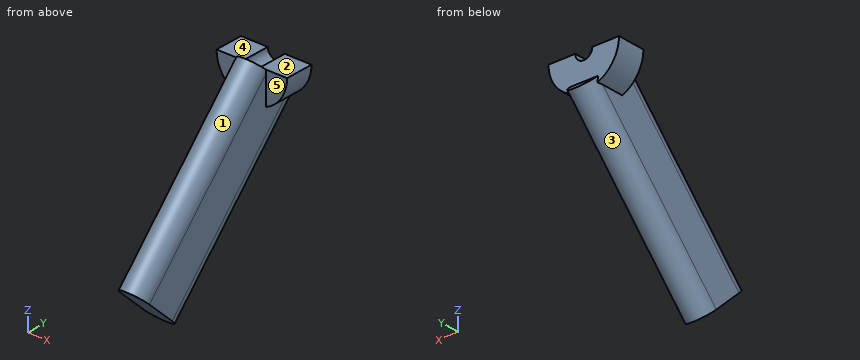
```python
from build123d import *

# Parameters (mm, degrees)
F1_DEPTH = 25
F5_DEPTH = 176


with BuildPart() as f1:
    # F0 (on Front) → F1 (new body)
    with BuildSketch(Plane.XZ):
        with BuildLine():
            ThreePointArc((-31, 0), (0, -31), (31, 0))
            Line((31, 0), (7.5, 0))
            ThreePointArc((7.5, 0), (0, -7.5), (-7.5, 0))
            Line((-7.5, 0), (-31, 0))
        make_face()
    extrude(amount=F1_DEPTH)

    # F4 (on face) → F5 (join)
    with BuildSketch(Plane(origin=(0, -11.816696451, -12.4813098776), x_dir=(1, 0, 0), z_dir=(0, -0.6875084422, -0.7261763849))):
        with BuildLine():
            Line((-12.5, 16), (0, 16))
            Line((0, 16), (12.5, 16))
            ThreePointArc((12.5, 16), (0, 28.5), (-12.5, 16))
        make_face()
        with BuildLine():
            Line((0, 16), (0, 3.5))
            ThreePointArc((0, 3.5), (8.8388347648, 7.1611652352), (12.5, 16))
            Line((12.5, 16), (0, 16))
        make_face()
        with BuildLine():
            ThreePointArc((-12.5, 16), (-8.8388347648, 7.1611652352), (0, 3.5))
            Line((0, 3.5), (0, 16))
            Line((0, 16), (-12.5, 16))
        make_face()
        with BuildLine():
            Line((0, -16), (0, -3.5))
            ThreePointArc((0, -3.5), (-8.8388347648, -7.1611652352), (-12.5, -16))
            ThreePointArc((-12.5, -16), (0, -28.5), (12.5, -16))
            Line((12.5, -16), (0, -16))
        make_face()
        with BuildLine():
            Line((0, 3.5), (0, 0))
            Line((0, 0), (0, -3.5))
            ThreePointArc((0, -3.5), (8.8388347648, -7.1611652352), (12.5, -16))
            Line((12.5, -16), (12.5, 16))
            ThreePointArc((12.5, 16), (8.8388347648, 7.1611652352), (0, 3.5))
        make_face()
        with BuildLine():
            Line((0, -3.5), (0, 0))
            Line((0, 0), (0, 3.5))
            ThreePointArc((0, 3.5), (-8.8388347648, 7.1611652352), (-12.5, 16))
            Line((-12.5, 16), (-12.5, -16))
            ThreePointArc((-12.5, -16), (-8.8388347648, -7.1611652352), (0, -3.5))
        make_face()
        with BuildLine():
            ThreePointArc((12.5, -16), (8.8388347648, -7.1611652352), (0, -3.5))
            Line((0, -3.5), (0, -16))
            Line((0, -16), (12.5, -16))
        make_face()
    extrude(amount=F5_DEPTH)


solid = f1.part
```
Could you check a few things on this model? Use its own coordinates, in mm. Face numbers are marked on the shaded views. A direction names the side the tool comes from. Round coordinates to 2 decimals unless told otherwise and drop trailing zeros. Loops run counter-clockwise (first coordinate to the right, second up) from the corner with the lowest first, then second, coordinate; pieces in that order, holes last. Notation, with made-up numbers: (32, -31) - (42, -31) arc R34 cw to (42, 8) - close; hole circle Ø8 at (56, 69.25). An arc over 180 degrees is marked (long way). Answer as CSV lines item,"result".
1. For pin 1 Ø8 at (x, y) = (-20, -97) entering from +Z; pin 2 Ø5 at (x, z) = (14, -17.5) entering from +Y; pin 3 Ø1 at (x, y) = (5, -107.5) entering from +Z; pin 4 Ø7 at (x, y) = (22, -8) entering from +Z, each with a flat end and sliding along its axis, tell me the tip position at first contact or that it passes through.
Filled in:
pin 1,"passes through"
pin 2,"stops at y = 0"
pin 3,"stops at z = -73"
pin 4,"stops at z = 0"
2. I want a section at A-A on x = 0. List the corners of the cut face in (y, z) for me.
Filled in:
outline,"(-153.51, -120.69) - (-112.12, -159.88) - (8.88, -32.08) - (0, -23.67) - (0, -7.5) - (-17.08, -7.5) - (-32.51, 7.11) - close"
3. On a 3-axis mill with a long thin cutter (end or side, diameter ignored), from which of +Z, -Z, +X, -X, +Y, -Y can I reach the whole of each face in a straight line? I mean the marked faces 1 and 2. Say none if no direction works.
Filled in:
face 1,"+Z, -Y"
face 2,"+Z, +X, -X, +Y"
4. I want a section at B-B on x = -26.5. List the corners of the cut face in (y, z) for me.
Filled in:
outline,"(-25, -16.09) - (0, -16.09) - (0, 0) - (-25, 0) - close"
5. Please list where these lines run through material, in increasing order: line 1 along X through (y, z) = (-126, -132.5); line 2 along Z through (x, y) = (-3.5, -130); line 3 along Z through (x, y) = (8, -5.5). Write a range as [from, to].
Filled in:
line 1,"x = [-12.5, 12.5]"
line 2,"z = [-142.96, -96.58]"
line 3,"z = [-43.05, 0]"
6. I want a section at C-C on x = -17.5. List the corners of the cut face in (y, z) for me, then the cut area to 3 significant figures.
Filled in:
outline,"(-25, -25.59) - (0, -25.59) - (0, 0) - (-25, 0) - close"
area,"640 mm^2"
7. We'd pull the mould along Z, two halves only. Please class the marked faces 3, 4 and 5: +Z half, -Z half, draft (parallel to the pull), parting line (faces both ways), or undercut.
Filled in:
face 3,"-Z half"
face 4,"+Z half"
face 5,"draft"
